Source: CAD feature listing. Evaluate the final solid. Frame: model axes, mm. A direction names the side the tool comes from. Give positions to 0.01 mm unless a question says otherwise; leave off trailing zeros. Write each loop counter-clockwise with the first axis right and the second up, starting at its lowest first coordinate (ties: lowest second). Pieces come first, ordered by that corner, then holes. Notation, with made-up numbers: (1, 78.25) - (32, 78.25) arc R12 cw to (32, 97.25) - close; hole circle Ø8 at (70, 19). An arc over 180 degrees is marked (long way). Answer as a JSON object with one key per item and string values. Group by question number.
from build123d import *

# Parameters (mm, degrees)
EXTRUDE_START       = 18
SKETCH_1_R          = 46
EXTRUDE_1_DEPTH     = 6
EXTRUDE_START_2     = 12
SKETCH_2_R          = 14
EXTRUDE_2_DEPTH     = 6
SKETCH_3_R          = 1.6
CUT_EXTRUDE_2_DEPTH = 89.746830929
SKETCH_4_R          = 5
CUT_EXTRUDE_4_DEPTH = 89.746830929


with BuildPart() as part:
    # 草图1 → 凸台-拉伸1 (new body)
    with BuildSketch(Plane.XY.offset(EXTRUDE_START)):
        with Locations((0, 26)):
            Circle(SKETCH_1_R)
    extrude(amount=EXTRUDE_1_DEPTH)

    # 草图2 → 凸台-拉伸2 (add)
    with BuildSketch(Plane.XY.offset(EXTRUDE_START_2)):
        with Locations((0, 26)):
            Circle(SKETCH_2_R)
    extrude(amount=EXTRUDE_2_DEPTH)

    # 草图3 → 切除-拉伸2 (cut, through all)
    with BuildSketch(Plane.XY):
        with Locations((24, 26)):
            Circle(SKETCH_3_R)
        with Locations((35, 35)):
            Circle(SKETCH_3_R)
        with Locations((35, 17)):
            Circle(SKETCH_3_R)
        with Locations((-12, 46.78)):
            Circle(SKETCH_3_R)
        with Locations((-25.29, 51.81)):
            Circle(SKETCH_3_R)
        with Locations((-9.71, 60.81)):
            Circle(SKETCH_3_R)
        with Locations((-12, 5.22)):
            Circle(SKETCH_3_R)
        with Locations((-9.71, -8.81)):
            Circle(SKETCH_3_R)
        with Locations((-25.29, 0)):
            Circle(SKETCH_3_R)
    extrude(amount=CUT_EXTRUDE_2_DEPTH, mode=Mode.SUBTRACT)

    # 草图4 → 切除-拉伸4 (cut, through all)
    with BuildSketch(Plane.XY):
        with Locations((0, 26)):
            Circle(SKETCH_4_R)
    extrude(amount=CUT_EXTRUDE_4_DEPTH, mode=Mode.SUBTRACT)


solid = part.part
Q1. Ray query, probe 1 along Y at (x, z) = (0.5, 23); probe 2 along Y at (x, z) = (35, 22.7); probe 3 along Y at (x, z) = (-24, 22). Return the intervals inside material, ascending. Write a range as [from, to].
Q2. Reachability of faces 4 (the flat face through (10, 37, 18)), 5 (the cylindrical face through (33.73, 34.03, 20.96)) from +Z, -Z, +X, -X, +Y, -Y: full face, straight path, thin tool, end or side. Return the list, or none.
Q3. Section D-D on x = -25.29. Return the cut outline in (y, z).
Q4. Section B-B on y = 51.81. Return the cut outline in (x, z), then the cut area to 3 significant figures.
Q5. Draft query along Y for faces 1 (the flat face through (0, 20, 12)), 2 (the cylindrical face through (-10.06, -10.37, 20.96)), 3 (the cylindrical face through (-5.99, 71.61, 20.96)). Return one class per face: released by +Y, released by -Y, zero draft, split by the parting line, or undercut.
Q6. Section C-C on z = 13.5. Return the cut outline in (x, y), then the cut area to 3 significant figures.
Q7. First-contact query: pin 1 Ø3 at (y, z) = (4, 17.5) entering from -X; pin 2 Ø5 at (x, y) = (35, 17) entering from -Z; pin 3 Ø6 at (y, z) = (15, 22.5) entering from +X. Flat tips, straight axial feed; report the tip coordinate or a pass-through.
Q8. Section A-A on x = 0. Return the cut outline in (y, z).
Taken from the geometry:
{
 "1": {"probe 1": "y = [-20, 21.03], [30.97, 72]", "probe 2": "y = [-3.85, 15.4], [18.6, 33.4], [36.6, 55.85]", "probe 3": "y = [-13.24, -0.95], [0.95, 50.86], [52.76, 65.24]"},
 "2": {"face 4": "-Z", "face 5": "+Z, -Z"},
 "3": {"outline": "(-12.42, 18) - (-1.6, 18) - (-1.6, 24) - (-12.42, 24) - close; (1.6, 18) - (50.21, 18) - (50.21, 24) - (1.6, 24) - close; (53.41, 18) - (64.42, 18) - (64.42, 24) - (53.41, 24) - close"},
 "4": {"outline": "(-38.08, 18) - (-26.89, 18) - (-26.89, 24) - (-38.08, 24) - close; (-23.69, 18) - (38.08, 18) - (38.08, 24) - (-23.69, 24) - close", "area": "438 mm²"},
 "5": {"face 1": "zero draft", "face 2": "undercut", "face 3": "split by the parting line"},
 "6": {"outline": "circle Ø28 at (0, 26); hole circle Ø10 at (0, 26)", "area": "537 mm²"},
 "7": {"pin 1": "stops at x = -41.14", "pin 2": "stops at z = 18", "pin 3": "stops at x = 45.3"},
 "8": {"outline": "(-20, 18) - (12, 18) - (12, 12) - (21, 12) - (21, 24) - (-20, 24) - close; (31, 12) - (40, 12) - (40, 18) - (72, 18) - (72, 24) - (31, 24) - close"}
}
